Drawing for the job (mm, zero at the part's lowest x, y, z). Coordinates: 2 decimals unless noted, no trailing zeros. Write each loop counter-clockwise with the first axis right and the second up, starting at its lowest first coordinate (ties: lowest second). Pieces come first, ordered by that corner, then holes. Notation, with made-up numbers: M 17.25,4 L 46.25,4 A19 ccw 46.25,25 Z; hole C 59,14.25 d5. An arc over 180 degrees is marked long. Use CSV: the item, a comma, the result in double quotes. Start each with the question number.
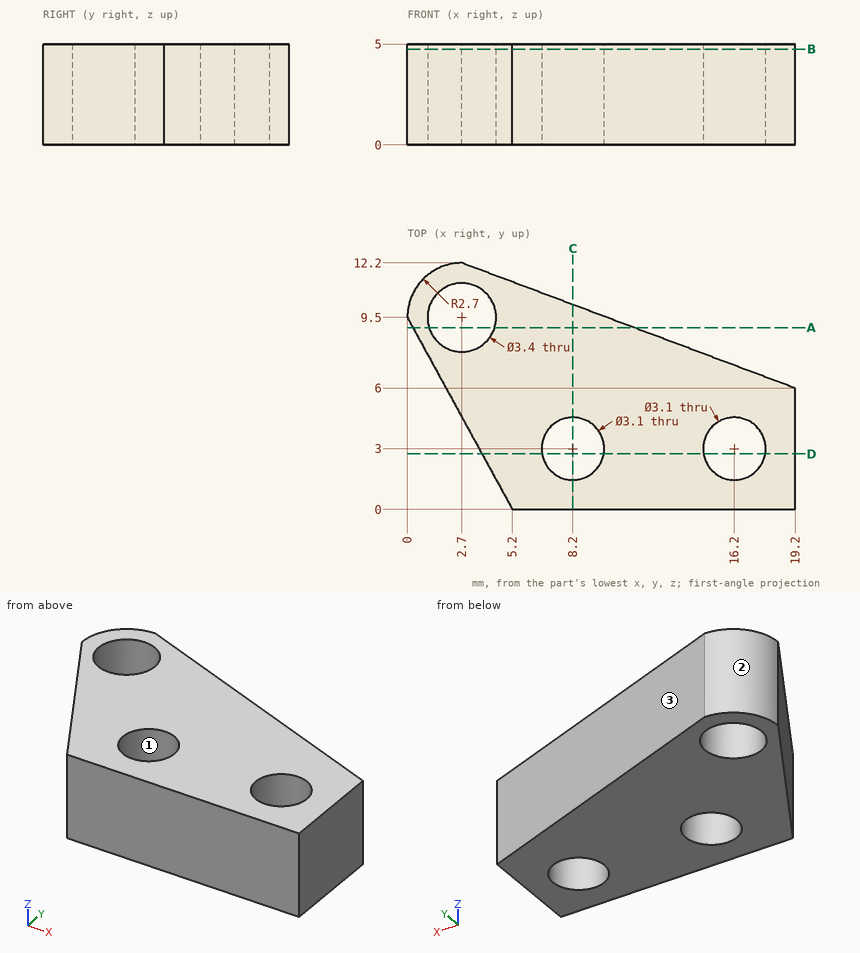
1) Wall check: L1, parallel to X at y = 2.5, z = 2.2; L2, parallel to X at y = 3.75, z = 1.2; L3, parallel to Y at x = 16.25, z = 3.85. Give the ranges that are in metal, low to high. Write a range as [from, to].
2) Band-saw the part on D-D on y = 2.75. List the corners of the cut face in (x, z), then the cut area to 3 significant figures.
3) Band-saw the part on B-B on z = 4.75. List the corners of the cut face in (x, y), then the cut area to 3 significant figures.
4) Band-saw the part on A-A on y = 9. List the corners of the cut face in (x, z), then the cut area to 3 significant figures.
5) Two-plate mould, pull along X, no slides. Class the marked faces 1, 2 and 3: pulls with the +X half, pulls with the -X half, needs draft (parallel to the pull), parting line crosses it, or undercut.
6) Band-saw the part on C-C on x = 8.2. List the corners of the cut face in (y, z), then the cut area to 3 significant figures.
7) Drop flat-ended pins along their axis: P1, Ø4, axis at x = 16.2, y = 3, coming from the +Z side; P2, Ø1, axis at x = 2, z = 3.5, coming from the +Y side; P3, Ø2.5, axis at x = 2.7, y = 9.5, coming from the +Z side; P4, Ø1, axis at x = 17, z = 1.5, coming from the +Y side. Give the stop position or say it passes through.
Findings below:
1,L1,"x = [3.83, 6.73], [9.67, 14.73], [17.67, 19.2]"
1,L2,"x = [3.15, 6.84], [9.56, 14.84], [17.56, 19.2]"
1,L3,"y = [0, 1.45], [4.55, 7.11]"
2,outline,"M 3.69,0 L 6.67,0 L 6.67,5 L 3.69,5 Z; M 9.73,0 L 14.67,0 L 14.67,5 L 9.73,5 Z; M 17.73,0 L 19.2,0 L 19.2,5 L 17.73,5 Z"
2,area,"46.9 mm2"
3,outline,"M 0,9.5 L 5.2,0 L 19.2,0 L 19.2,6 L 2.7,12.2 A2.7 ccw Z; hole C 2.7,9.5 d3.4; hole C 8.2,3 d3.1; hole C 16.2,3 d3.1"
3,area,"133 mm2"
4,outline,"M 0.27,0 L 1.08,0 L 1.08,5 L 0.27,5 Z; M 4.32,0 L 11.22,0 L 11.22,5 L 4.32,5 Z"
4,area,"38.5 mm2"
5,face 1,"undercut"
5,face 2,"pulls with the -X half"
5,face 3,"pulls with the +X half"
6,outline,"M 0,0 L 1.45,0 L 1.45,5 L 0,5 Z; M 4.55,0 L 10.13,0 L 10.13,5 L 4.55,5 Z"
6,area,"35.2 mm2"
7,P1,"stops at z = 5"
7,P2,"stops at y = 12.19"
7,P3,"passes through"
7,P4,"stops at y = 7.01"
